Work out the finished part from the listing and answer in its coordinate system (mm). A direction names the side the tool comes from. Round coordinates to 2 decimals unless told otherwise and drop trailing zeros. Order: outer loops, then holes, each group sorted by start corner. A loop starts at its lowest first (then second) coordinate and runs counter-clockwise, first axis right, second up. Notation, with made-up numbers: (82, 19) - (141, 19) arc R10 ccw to (141, 36) - close; hole circle Ø11 at (4.5, 89). An arc over 180 degrees is marked (long way). One line per question, with ' | ' between items. Start each with the question number.
from build123d import *

# Parameters (mm, degrees)
Y_KSEKLIK_EKSTR_ZYON1_DEPTH = 77.5
KES_EKSTR_ZYON1_START       = 7.992125884
KES_EKSTR_ZYON1_OUTLINE_R   = 3
KES_EKSTR_ZYON1_DEPTH       = 9.5000001


# Read off the part's stored shape, not the designer's step: Kes-Ekstrüzyon1
with BuildPart() as part:
    # Çizim1 → Yükseklik-Ekstrüzyon1 (new body)
    with BuildSketch(Plane.XY):
        Polygon((-33.046021585, 17.492125984), (29.953978415, 17.492125984), (29.953978415, 11.492125984), (25.453978415, 11.492125984), (15.453978415, 1.492125984), (15.453978415, -8.507874016), (8.453978415, -8.507874016), (8.453978415, 7.492125984), (-11.546021585, 7.492125984), (-11.546021585, -8.507874016), (-18.546021585, -8.507874016), (-18.546021585, 1.492125984), (-28.546021585, 11.492125984), (-33.046021585, 11.492125984), align=None)
    extrude(amount=Y_KSEKLIK_EKSTR_ZYON1_DEPTH)

    # Kes-Ekstrüzyon1 outline → Kes-Ekstrüzyon1 (cut)
    with BuildSketch(Plane(origin=(0, 0, 0), x_dir=(1, 0, 0), z_dir=(0, 1, 0)).offset(KES_EKSTR_ZYON1_START)):
        with Locations((-28.046021585, -13.5)):
            Circle(KES_EKSTR_ZYON1_OUTLINE_R)
        with Locations((24.953978415, -64)):
            Circle(KES_EKSTR_ZYON1_OUTLINE_R)
        with Locations((-28.046021585, -64)):
            Circle(KES_EKSTR_ZYON1_OUTLINE_R)
        with Locations((24.953978415, -13.5)):
            Circle(KES_EKSTR_ZYON1_OUTLINE_R)
    extrude(amount=KES_EKSTR_ZYON1_DEPTH, mode=Mode.SUBTRACT)


solid = part.part
1) Straight lines are drawn through the part: line 1 (X direction, y = 13.5, z = 13.5); line 2 (X direction, y = -0.25, z = 5); line 3 (Y direction, x = -3.5, z = 57). For each, find the intervals that lie inside material, in ascending order.
2) Section B-B on z = 13.5 is taken. Give the vertices of the cut face in (x, y).
3) For faces 5 (the flat face through (15.454, -3, 38)), 6 (the flat face through (-18.546, -4, 38)), 7 (the flat face through (8.454, -1, 38)), determine the directions among +Z, -Z, +X, -X, +Y, -Y from which every point of the face is accessible in a straight line to the end or side of a thin tool.
4) Flat-ended cylindrical pins translate along their axes: pin 1 (8 mm diameter, centred on y = 5, z = 49, fed in from +X); pin 2 (5 mm diameter, centred on y = -3, z = 42, fed in from -X); pin 3 (1.5 mm diameter, centred on x = -8.5, z = 65, fed in from -Y); pin 4 (3.5 mm diameter, centred on x = -28.05, z = 13.5, fed in from +Y). Find the tip coordinate at first contact, or state that the pin passes through.
5) Section D-D on y = 3.75 is taken. Give the vertices of the cut face in (x, z).
6) Section C-C on x = -27 is taken. Give the vertices of the cut face in (y, z).
7) Determine the mould class of faces 1 (the flat face through (28, 11.492, 38)), 2 (the flat face through (-23.476, 6.422, 38.207)), 3 (the cylindrical face through (21.957, 13.731, 13.368)), 4 (the cylindrical face through (21.957, 13.731, 63.868)) for opening direction X: released by +X, released by -X, zero draft, split by the parting line, or undercut.
8) Section A-A on y = 14.5 is taken. Give the vertices of the cut face in (x, z), and give its area (3 significant figures).
Recorded:
1) line 1: x = -33.05 to -31.05, -25.05 to 21.95, 27.95 to 29.95 | line 2: x = -18.55 to -11.55, 8.45 to 15.45 | line 3: y = 7.49 to 17.49
2) outline: (-33.05, 11.49) - (-31.05, 11.49) - (-31.05, 17.49) - (-33.05, 17.49) - close; (-25.05, 7.99) - (-18.55, 1.49) - (-18.55, -8.51) - (-11.55, -8.51) - (-11.55, 7.49) - (8.45, 7.49) - (8.45, -8.51) - (15.45, -8.51) - (15.45, 1.49) - (21.95, 7.99) - (21.95, 17.49) - (-25.05, 17.49) - close; (27.95, 11.49) - (29.95, 11.49) - (29.95, 17.49) - (27.95, 17.49) - close
3) face 5: +Z, -Z, +X, -Y | face 6: +Z, -Z, -X, -Y | face 7: +Z, -Z, -Y
4) pin 1: stops at x = 22.96 | pin 2: stops at x = -18.55 | pin 3: stops at y = 7.49 | pin 4: passes through
5) outline: (-20.8, 0) - (-11.55, 0) - (-11.55, 77.5) - (-20.8, 77.5) - close; (8.45, 0) - (17.71, 0) - (17.71, 77.5) - (8.45, 77.5) - close
6) outline: (9.95, 0) - (17.49, 0) - (17.49, 10.69) - (9.95, 10.69) - close; (9.95, 16.31) - (17.49, 16.31) - (17.49, 61.19) - (9.95, 61.19) - close; (9.95, 66.81) - (17.49, 66.81) - (17.49, 77.5) - (9.95, 77.5) - close
7) face 1: zero draft | face 2: released by -X | face 3: undercut | face 4: undercut
8) outline: (-33.05, 0) - (29.95, 0) - (29.95, 77.5) - (-33.05, 77.5) - close; hole circle Ø6 at (-28.05, 13.5); hole circle Ø6 at (-28.05, 64); hole circle Ø6 at (24.95, 13.5); hole circle Ø6 at (24.95, 64) | area: 4,770 mm²
